Can you work these out from the model? Positions are in its coordinate system, mm. Round coordinates to 2 decimals unless told otherwise and drop trailing zeros. Loops run counter-clockwise (first coordinate to the right, second up) from the corner with the lowest first, then second, coordinate; pieces in that order, holes last. Notation, with made-up numbers: M 87,48.25 L 92,48.25 A16 cw 92,66.25 Z; hole C -13,-2.5 d2. An arc over 180 degrees is marked long. Return JSON: item names as keys, results as strings.
```python
from build123d import *

# Parameters (mm, degrees)
F1_DEPTH = 700
F2_DEPTH = 45
F3_R     = 0.7


with BuildPart() as f1:
    # F0 (on Front) → F1 (new body)
    with BuildSketch(Plane.XZ):
        with BuildLine():
            ThreePointArc((8.660254, -5), (9.659258, -2.58819), (10, 0))
            ThreePointArc((10, 0), (9.659258, 2.588191), (8.660254, 5))
            ThreePointArc((8.660254, 5), (5, 8.660254), (0, 10))
            ThreePointArc((0, 10), (-5, 8.660254), (-8.660254, 5))
            ThreePointArc((-8.660254, 5), (-10, 0), (-8.660254, -5))
            ThreePointArc((-8.660254, -5), (-5, -8.660254), (0, -10))
            ThreePointArc((0, -10), (5, -8.660254), (8.660254, -5))
        make_face()
    extrude(amount=F1_DEPTH)

    # F0 (on Front) → F2 (join)
    with BuildSketch(Plane.XZ):
        with BuildLine():
            ThreePointArc((8.660254, 5), (9.659258, 2.588191), (10, 0))
            ThreePointArc((10, 0), (9.659258, -2.58819), (8.660254, -5))
            ThreePointArc((8.660254, -5), (11.296935, -2.795508), (14.733726, -2.813771))
            ThreePointArc((14.733726, -2.813771), (15, 0), (14.733726, 2.813771))
            ThreePointArc((14.733726, 2.813771), (11.296935, 2.795509), (8.660254, 5))
        make_face()
        with BuildLine():
            ThreePointArc((0, 10), (5, 8.660254), (8.660254, 5))
            ThreePointArc((8.660254, 5), (8.069449, 8.385679), (9.80366, 11.352896))
            ThreePointArc((9.80366, 11.352896), (7.5, 12.990381), (4.930066, 14.166667))
            ThreePointArc((4.930066, 14.166667), (3.227486, 11.181187), (0, 10))
        make_face()
        with BuildLine():
            ThreePointArc((9.80366, -11.352896), (8.069449, -8.385678), (8.660254, -5))
            ThreePointArc((8.660254, -5), (5, -8.660254), (0, -10))
            ThreePointArc((0, -10), (3.227486, -11.181187), (4.930066, -14.166667))
            ThreePointArc((4.930066, -14.166667), (7.5, -12.990381), (9.80366, -11.352896))
        make_face()
        with BuildLine():
            ThreePointArc((-8.660254, 5), (-5, 8.660254), (0, 10))
            ThreePointArc((0, 10), (-3.227486, 11.181187), (-4.930066, 14.166667))
            ThreePointArc((-4.930066, 14.166667), (-7.5, 12.990381), (-9.80366, 11.352896))
            ThreePointArc((-9.80366, 11.352896), (-8.069449, 8.385678), (-8.660254, 5))
        make_face()
        with BuildLine():
            ThreePointArc((-4.930066, -14.166667), (-3.227486, -11.181187), (0, -10))
            ThreePointArc((0, -10), (-5, -8.660254), (-8.660254, -5))
            ThreePointArc((-8.660254, -5), (-8.069449, -8.385678), (-9.80366, -11.352896))
            ThreePointArc((-9.80366, -11.352896), (-7.5, -12.990381), (-4.930066, -14.166667))
        make_face()
        with BuildLine():
            ThreePointArc((-8.660254, -5), (-10, 0), (-8.660254, 5))
            ThreePointArc((-8.660254, 5), (-11.296935, 2.795508), (-14.733726, 2.813771))
            ThreePointArc((-14.733726, 2.813771), (-15, 0), (-14.733726, -2.813771))
            ThreePointArc((-14.733726, -2.813771), (-11.296935, -2.795508), (-8.660254, -5))
        make_face()
    extrude(amount=F2_DEPTH)

    # F3
    f3_edges = [f1.edges().sort_by_distance(p)[0] for p in [
        (14.733726, -22.5, -2.813771),
        (9.80366, -22.5, -11.352896),
        (4.930066, -22.5, -14.166667),
        (-4.930066, -22.5, -14.166667),
        (-9.80366, -22.5, -11.352896),
        (-14.733726, -22.5, -2.813771),
        (-14.733726, -22.5, 2.813771),
        (-9.80366, -22.5, 11.352896),
        (-4.930066, -22.5, 14.166667),
        (4.930066, -22.5, 14.166667),
        (9.80366, -22.5, 11.352896),
        (14.733726, -22.5, 2.813771),
    ]]
    fillet(f3_edges, radius=F3_R)


solid = f1.part
```
Q1. I'm going to push flat-ended pins straight in: pin 1 Ø8 at (x, y) = (8.5, -367.5) entering from -Z; pin 2 Ø3 at (x, y) = (2.5, -548.5) entering from +Z; pin 3 Ø5 at (x, z) = (-13, -2) entering from -Y. Where does each tip first touch, or does it pass through?
Results:
{"pin 1": "stops at z = -8.93", "pin 2": "stops at z = 9.95", "pin 3": "stops at y = -45"}
Q2. If I drill on line 1 along Z through (x, y) = (-5, -479.5); line 2 along Z through (x, y) = (1.5, -171.5); line 3 along X through (y, z) = (-102, 3), over which ranges is the centre line in solid material (lowest first)?
Results:
{"line 1": "z = -8.66 to 8.66", "line 2": "z = -9.89 to 9.89", "line 3": "x = -9.54 to 9.54"}
Q3. Suppose I cut it at A-A, the plane y = -62. Please give me the cut outline in (x, z), plus the area to 3 significant figures.
Results:
{"outline": "M 8.66,-5 A10 ccw 10,0 A10 ccw 8.66,5 A10 ccw long Z", "area": "314 mm2"}
